from build123d import *

# Parameters (mm, degrees)
SKETCH1_R           = 1.5
BOSS_EXTRUDE1_DEPTH = 2
SKETCH2_R           = 1.5
BOSS_EXTRUDE2_DEPTH = 2
FILLET1_R           = 1


with BuildPart() as part:
    # Sketch1 → Boss-Extrude1 (new body)
    with BuildSketch(Plane.XY):
        with BuildLine():
            Line((0, 96), (0, 0))
            Line((0, 0), (10.5, 0))
            Line((10.5, 0), (10.5, -2))
            Line((10.5, -2), (24.5, -2))
            Line((24.5, -2), (24.5, 0))
            Line((24.5, 0), (28, 0))
            Line((28, 0), (28, 7))
            ThreePointArc((28, 7), (26.535533906, 10.535533906), (23, 12))
            Line((23, 12), (17, 12))
            ThreePointArc((17, 12), (13.464466094, 13.464466094), (12, 17))
            Line((12, 17), (12, 79))
            ThreePointArc((12, 79), (13.464466094, 82.535533906), (17, 84))
            Line((17, 84), (23, 84))
            ThreePointArc((23, 84), (26.535533906, 85.464466094), (28, 89))
            Line((28, 89), (28, 96))
            Line((28, 96), (24.5, 96))
            Line((24.5, 96), (24.5, 98))
            Line((24.5, 98), (10.5, 98))
            Line((10.5, 98), (10.5, 96))
            Line((10.5, 96), (0, 96))
        make_face()
        with Locations((20.5, 2.5)):
            Circle(SKETCH1_R, mode=Mode.SUBTRACT)
        with Locations((20.5, 93.5)):
            Circle(SKETCH1_R, mode=Mode.SUBTRACT)
    extrude(amount=BOSS_EXTRUDE1_DEPTH)

    # Sketch2 → Boss-Extrude2 (add)
    with BuildSketch(Plane.ZY):
        with BuildLine():
            Line((0, 96), (-8.5, 96))
            Line((-8.5, 96), (-8.5, 98))
            Line((-8.5, 98), (-22.5, 98))
            Line((-22.5, 98), (-22.5, 96))
            Line((-22.5, 96), (-26, 96))
            Line((-26, 96), (-26, 89))
            ThreePointArc((-26, 89), (-24.535533906, 85.464466094), (-21, 84))
            Line((-21, 84), (-15, 84))
            ThreePointArc((-15, 84), (-11.464466094, 82.535533906), (-10, 79))
            Line((-10, 79), (-10, 17))
            ThreePointArc((-10, 17), (-11.464466094, 13.464466094), (-15, 12))
            Line((-15, 12), (-21, 12))
            ThreePointArc((-21, 12), (-24.535533906, 10.535533906), (-26, 7))
            Line((-26, 7), (-26, 0))
            Line((-26, 0), (-22.5, 0))
            Line((-22.5, 0), (-22.5, -2))
            Line((-22.5, -2), (-8.5, -2))
            Line((-8.5, -2), (-8.5, 0))
            Line((-8.5, 0), (0, 0))
            Line((0, 0), (0, 96))
        make_face()
        with Locations((-18.5, 93.5)):
            Circle(SKETCH2_R, mode=Mode.SUBTRACT)
        with Locations((-18.5, 2.5)):
            Circle(SKETCH2_R, mode=Mode.SUBTRACT)
    extrude(amount=-BOSS_EXTRUDE2_DEPTH)

    # Fillet1
    fillet1_edges = [part.edges().sort_by_distance(p)[0] for p in [
        (0, 48, 2),
    ]]
    fillet(fillet1_edges, radius=FILLET1_R)


solid = part.part
Input: part model. Units: mm. Frame: model coordinates. A direction names the side the tool comes from. Coordinates: 2 decimals unless noted, no trailing zeros. Write each loop counter-clockwise with the first axis right and the second up, starting at its lowest first coordinate (ties: lowest second). Pieces come first, ordered by that corner, then holes. Notation, with made-up numbers: M -31,-2.75 L -3,-2.75 A33 cw -3,36.25 Z; hole C -20.75,25 d1. An arc over 180 degrees is marked long. Answer as a JSON object with one key per item and string values. Group by question number.
(1) Set-up query: faces 4 (the face through (9, 49, 0)), 5 (the face through (1.7, 96, -0.8)), 6 (the face through (1, 97, -22.5)), 7 (the face through (1, 11, -24)), 8 (the face through (1, -1, -22.5)). Return all of +Z, -Z, +X, -X, +Y, -Y with unobstructed straight access to the full face (end or side cutting, diameter ignored); none if empty.
(2) Section C-C on z = -18.5. Output: boundary loops of the cut face in (x, y), plus the area to 3 significant figures.
(3) Ray query, line 1 along Y through (x, z) = (0.8, -18.5); line 2 along Z through (x, y) = (1.55, 93.5); line 3 along X through (y, z) = (93.5, 1.1). Return the intervals inside material, ascending. Write a range as [from, to].
(4) Contact query for flat-ended pins moving along their axis: P1, Ø1, axis at x = 27, z = 0.5, coming from the -Y side; P2, Ø10, axis at x = 13, y = 21, coming from the -Z side; P3, Ø0.6, axis at y = -0.5, z = 0.5, coming from the +X side; P4, Ø1.8, axis at x = 20.5, y = 2.5, coming from the -Z side. Output: stop coordinate, or through.
(5) Mould query, pull axis X, two halves, no side actions, for faces 1 (the face through (12, 48, 1)), 2 (the face through (1, -1, -8.5)), 3 (the face through (19, 2.57, 0.99)). Classes: pulls with the +X half, pulls with the -X half, needs draft (parallel to the pull), parting line crosses it, or undercut.
(6) Section A-A on x = 20.5. Output: boundary loops of the cut face in (y, z), plus the area to 3 significant figures.
(7) Section D-D on y = 83. Output: boundary loops of the cut face in (x, z).
(8) Section B-B on y = 2.5. Output: boundary loops of the cut face in (x, z), plus the area to 3 significant figures.
Result set:
{
 "1": {"face 4": "-Z, +X, +Y, -Y", "face 5": "+Z, -X, +Y", "face 6": "-Z, +X, -X, +Y", "face 7": "-Z, +X, -X", "face 8": "-Z, +X, -X, -Y"},
 "2": {"outline": "M 0,-2 L 2,-2 L 2,1 L 0,1 Z; M 0,4 L 2,4 L 2,12 L 0,12 Z; M 0,84 L 2,84 L 2,92 L 0,92 Z; M 0,95 L 2,95 L 2,98 L 0,98 Z", "area": "44.0 mm2"},
 "3": {"line 1": "y = [-2, 1], [4, 12], [84, 92], [95, 98]", "line 2": "z = [-26, -20], [-17, 2]", "line 3": "x = [0.01, 19], [22, 28]"},
 "4": {"P1": "stops at y = 0", "P2": "stops at z = 0", "P3": "stops at x = 24.5", "P4": "passes through"},
 "5": {"face 1": "pulls with the +X half", "face 2": "needs draft", "face 3": "undercut"},
 "6": {"outline": "M -2,0 L 1,0 L 1,2 L -2,2 Z; M 4,0 L 12,0 L 12,2 L 4,2 Z; M 84,0 L 92,0 L 92,2 L 84,2 Z; M 95,0 L 98,0 L 98,2 L 95,2 Z", "area": "44.0 mm2"},
 "7": {"outline": "M 0,-12 L 2,-12 L 2,0 L 14,0 L 14,2 L 1,2 A1 ccw 0,1 Z"},
 "8": {"outline": "M 0,-26 L 2,-26 L 2,-20 L 0,-20 Z; M 0,-17 L 2,-17 L 2,0 L 19,0 L 19,2 L 1,2 A1 ccw 0,1 Z; M 22,0 L 28,0 L 28,2 L 22,2 Z", "area": "95.8 mm2"}
}
